```python
from build123d import *

# Parameters (mm, degrees)
SKETCH1_R           = 4.862500054
SKETCH1_W           = 76.454
SKETCH1_H           = 38.354
BOSS_EXTRUDE1_DEPTH = 50.8
BOSS_EXTRUDE2_DEPTH = 5.08
BOSS_EXTRUDE3_DEPTH = 55.88
SKETCH4_R           = 3.429
CUT_EXTRUDE1_DEPTH  = 50.8
SKETCH5_R           = 3.81
CUT_EXTRUDE2_DEPTH  = 50.8
SKETCH6_R           = 5.08
CUT_EXTRUDE3_DEPTH  = 50.8


with BuildPart() as part:
    # Sketch1 → Boss-Extrude1 (new body)
    with BuildSketch(Plane.XY):
        with BuildLine():
            Line((-43.029964919, -17.522331458), (-43.029964919, 19.177))
            Line((-43.029964919, 19.177), (-43.029964919, 49.89109769))
            ThreePointArc((-43.029964919, 49.89109769), (-33.369881409, 59.115507734), (-23.699543278, 49.901848605))
            Line((-23.699543278, 49.901848605), (0, 24.257))
            Line((0, 24.257), (23.699543278, 49.901848605))
            ThreePointArc((23.699543278, 49.901848605), (33.369881409, 59.115507734), (43.029964919, 49.89109769))
            Line((43.029964919, 49.89109769), (43.029964919, 19.177))
            Line((43.029964919, 19.177), (43.029964919, -17.522331458))
            Line((43.029964919, -17.522331458), (63.5, -44.577))
            Line((63.5, -44.577), (-63.5, -44.577))
            Line((-63.5, -44.577), (-43.029964919, -17.522331458))
        make_face()
        with Locations((-33.364499946, 49.439500054)):
            Circle(SKETCH1_R, mode=Mode.SUBTRACT)
        with Locations(Location((33.364499946, 49.439500054, 0), (0, 0, 180))):
            Circle(SKETCH1_R, mode=Mode.SUBTRACT)
        Rectangle(SKETCH1_W, SKETCH1_H, mode=Mode.SUBTRACT)
    extrude(amount=BOSS_EXTRUDE1_DEPTH)

    # Sketch2 → Boss-Extrude2 (add)
    with BuildSketch(Plane(origin=(0, 0, 0), x_dir=(-1, 0, 0), z_dir=(0, 0, -1))):
        with BuildLine():
            Line((-43.029964919, 49.89109769), (-43.029964919, -17.522331458))
            Line((-43.029964919, -17.522331458), (-63.5, -44.577))
            Line((-63.5, -44.577), (63.5, -44.577))
            Line((63.5, -44.577), (43.029964919, -17.522331458))
            Line((43.029964919, -17.522331458), (43.029964919, 49.89109769))
            ThreePointArc((43.029964919, 49.89109769), (33.370126568, 59.556310005), (23.699543278, 49.901848605))
            Line((23.699543278, 49.901848605), (0, 24.257))
            Line((0, 24.257), (-23.699543278, 49.901848605))
            ThreePointArc((-23.699543278, 49.901848605), (-33.370126568, 59.556310005), (-43.029964919, 49.89109769))
        make_face()
    extrude(amount=BOSS_EXTRUDE2_DEPTH)

    # Sketch3 → Boss-Extrude3 (add)
    with BuildSketch(Plane(origin=(0, 0, -5.08), x_dir=(-1, 0, 0), z_dir=(0, 0, -1))):
        with BuildLine():
            Line((-33.370126568, 59.556310005), (33.370126568, 59.556310005))
            ThreePointArc((33.370126568, 59.556310005), (26.537689117, 56.729560126), (23.699543278, 49.901848605))
            Line((23.699543278, 49.901848605), (0, 24.257))
            Line((0, 24.257), (-23.699543278, 49.901848605))
            ThreePointArc((-23.699543278, 49.901848605), (-26.537689117, 56.729560126), (-33.370126568, 59.556310005))
        make_face()
    extrude(amount=-BOSS_EXTRUDE3_DEPTH)

    # Sketch4 → Cut-Extrude1 (cut)
    with BuildSketch(Plane.XY.offset(50.8)):
        with Locations((-0.569554056, 49.439500054)):
            Circle(SKETCH4_R)
    extrude(amount=-CUT_EXTRUDE1_DEPTH, mode=Mode.SUBTRACT)

    # Sketch5 → Cut-Extrude2 (cut)
    with BuildSketch(Plane.XY.offset(50.8)):
        with Locations((-0.569554056, 49.439500054)):
            Circle(SKETCH5_R)
    extrude(amount=-CUT_EXTRUDE2_DEPTH, mode=Mode.SUBTRACT)

    # Sketch6 → Cut-Extrude3 (cut)
    with BuildSketch(Plane.XY.offset(50.8)):
        with Locations((-33.364499946, 49.439500054)):
            Circle(SKETCH6_R)
        with Locations((33.364499946, 49.439500054)):
            Circle(SKETCH6_R)
    extrude(amount=-CUT_EXTRUDE3_DEPTH, mode=Mode.SUBTRACT)


solid = part.part
```
CAD build for the part. Positions are in the model's coordinates, mm. A direction names the side the tool comes from. Coordinates: 2 decimals unless noted, no trailing zeros. Order: outer loops, then holes, each group sorted by start corner. A loop starts at its lowest first (then second) coordinate and runs counter-clockwise, first axis right, second up.
(1) Mould opens along Y. For faces 4 (the face through (-40.272, 56.652, -2.504)), 5 (the face through (38.227, 0, 25)), 6 (the face through (1, 8, -5.08)) say: released by +Y, released by -Y, zero draft, split by the parting line, or undercut.
Solution:
face 4: released by +Y
face 5: undercut
face 6: zero draft
(2) Saw through at D-D, the plane y = 33.5. Write the cut outline in (x, z), and give its area (3 significant figures).
Solution:
outline: (-43.03, -5.08) - (43.03, -5.08) - (43.03, 50.8) - (-43.03, 50.8) - close
area: 4,810 mm2
(3) Which spindle directions (+Z, -Z, +X, -X, +Y, -Y) get a long thin tool onto all of the face, cutting with end or side? Do faces 1 (the face through (1, 0, 0)), 2 (the face through (-43.03, 16, 23)), 3 (the face through (0, 59.556, 22)). Say none if no direction does.
Solution:
face 1: +Z
face 2: +Z, -Z, -X, +Y
face 3: +Z, -Z, +X, -X, +Y
(4) Saw through at C-C, the plane z = 11. Write the cut outline in (x, y).
Solution:
outline: (-63.5, -44.58) - (63.5, -44.58) - (43.03, -17.52) - (43.03, 49.89) arc R9.68 ccw to (23.7, 49.9) arc R9.67 cw to (33.37, 59.56) - (-33.37, 59.56) arc R9.67 cw to (-23.7, 49.9) arc R9.68 ccw to (-43.03, 49.89) - (-43.03, -17.52) - close; hole circle Ø10.16 at (-33.36, 49.44); hole (-38.23, -19.18) - (38.23, -19.18) - (38.23, 19.18) - (-38.23, 19.18) - close; hole circle Ø7.62 at (-0.57, 49.44); hole circle Ø10.16 at (33.36, 49.44)
(5) Saw through at B-B, the plane x = -9.5. Write the cut outline in (y, z), and give its area (3 significant figures).
Solution:
outline: (-44.58, -5.08) - (59.56, -5.08) - (59.56, 50.8) - (19.18, 50.8) - (19.18, 0) - (-19.18, 0) - (-19.18, 50.8) - (-44.58, 50.8) - close
area: 3,870 mm2
(6) Pin check, flat tips, straight feed: pin 1 Ø1.5 at (y, z) = (15, 18) entering from -X; pin 2 Ø4 at (x, y) = (0, 49) entering from +Z; pin 3 Ø17 at (y, z) = (6.5, 33.5) entering from +X. Stop position of each tip, or through.
Solution:
pin 1: stops at x = -43.03
pin 2: stops at z = 0
pin 3: stops at x = 43.03
(7) Drill centre lines: L1, parallel to X at y = -15, z = 0.5; L2, parallel to Y at x = 3.5, z = 6; L3, parallel to Y at x = 0.5, z = 9. Where is each one in solid material? Low to high.
Solution:
L1: x = -43.03 to -38.23, 38.23 to 43.03
L2: y = -44.58 to -19.18, 19.18 to 59.56
L3: y = -44.58 to -19.18, 19.18 to 45.78, 53.1 to 59.56
(8) Saw through at A-A, the plane y = 1.5. Write the cut outline in (x, z).
Solution:
outline: (-43.03, -5.08) - (43.03, -5.08) - (43.03, 50.8) - (38.23, 50.8) - (38.23, 0) - (-38.23, 0) - (-38.23, 50.8) - (-43.03, 50.8) - close
